Check sheet for the modelled part. Datum: model origin and axes. Units: mm. Round coordinates to 2 decimals unless told otherwise and drop trailing zeros. Order: outer loops, then holes, each group sorted by start corner. A loop starts at its lowest first (then second) coordinate and runs counter-clockwise, first axis right, second up. Notation, with made-up numbers: (65.25, 54.25) -> (103.25, 54.25) arc R33 ccw to (103.25, 88.25) -> close; hole circle Ø4 at (74.25, -32). An arc over 180 degrees is marked (long way). Answer in a Markdown table with one row per item.
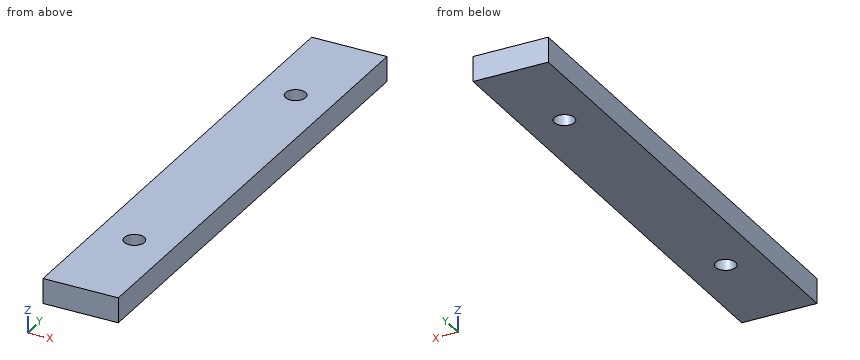
from build123d import *

# Parameters (mm, degrees)
F0_W     = 38.1
F0_H     = 254
F1_DEPTH = 12.7
F3_D     = 10.16


with BuildPart() as f1:
    # F0 (on Top) → F1 (new body)
    with BuildSketch(Plane.XY):
        Rectangle(F0_W, F0_H)
    extrude(amount=-F1_DEPTH)

    # F3 (through all)
    with Locations(Plane.XY):
        with Locations((0, 76.2), (0, -76.2)):
            Hole(F3_D / 2)


solid = f1.part
Item 1: Cross-section at A-A (x = 0). Record the boundary of the cut face in (y, z).
Result sheet:
| item | result |
|---|---|
| outline | (-127, -12.7) -> (-81.28, -12.7) -> (-81.28, 0) -> (-127, 0) -> close; (-71.12, -12.7) -> (71.12, -12.7) -> (71.12, 0) -> (-71.12, 0) -> close; (81.28, -12.7) -> (127, -12.7) -> (127, 0) -> (81.28, 0) -> close |
Item 2: Cross-section at C-C (z = -10). Record the boundary of the cut face in (x, y).
Result sheet:
| item | result |
|---|---|
| outline | (-19.05, -127) -> (19.05, -127) -> (19.05, 127) -> (-19.05, 127) -> close; hole circle Ø10.16 at (0, -76.2); hole circle Ø10.16 at (0, 76.2) |
Item 3: Scan lines: line 1 (Y direction, x = 0, z = -10); line 2 (Y direction, x = 1, z = -5.75). Record each from-to range of solid material in increasing order. Write a range as [from, to].
Result sheet:
| item | result |
|---|---|
| line 1 | y = [-127, -81.28], [-71.12, 71.12], [81.28, 127] |
| line 2 | y = [-127, -81.18], [-71.22, 71.22], [81.18, 127] |
Item 4: Cross-section at B-B (y = -76.2). Record the boundary of the cut face in (x, z), and give its area (3 significant figures).
Result sheet:
| item | result |
|---|---|
| outline | (-19.05, -12.7) -> (-5.08, -12.7) -> (-5.08, 0) -> (-19.05, 0) -> close; (5.08, -12.7) -> (19.05, -12.7) -> (19.05, 0) -> (5.08, 0) -> close |
| area | 355 mm^2 |
